```python
from build123d import *

# Parameters (mm, degrees)
SKETCH1_W           = 31.75
SKETCH1_H           = 7.9375
BOSS_EXTRUDE1_DEPTH = 3.175
SKETCH2_R           = 2.38125
BOSS_EXTRUDE2_DEPTH = 1.5875
SHELL1_T            = -1.5875
SKETCH3_R           = 1.5875
SKETCH3_R_2         = 0.79375
BOSS_EXTRUDE4_DEPTH = 1.397


with BuildPart() as part:
    # Sketch1 → Boss-Extrude1 (new body)
    with BuildSketch(Plane(origin=(0, 0, 0), x_dir=(1, 0, 0), z_dir=(0, 1, 0))):
        with Locations((15.875, 3.96875)):
            Rectangle(SKETCH1_W, SKETCH1_H)
    extrude(amount=BOSS_EXTRUDE1_DEPTH)

    # Sketch2 → Boss-Extrude2 (add)
    with BuildSketch(Plane(origin=(0, 3.175, 0), x_dir=(1, 0, 0), z_dir=(0, 1, 0))):
        with Locations((3.96875, 3.96875)):
            Circle(SKETCH2_R)
        with Locations((11.90625, 3.96875)):
            Circle(SKETCH2_R)
        with Locations((19.84375, 3.96875)):
            Circle(SKETCH2_R)
        with Locations((27.78125, 3.96875)):
            Circle(SKETCH2_R)
    extrude(amount=BOSS_EXTRUDE2_DEPTH)

    # Shell1
    shell1_openings = [part.faces().sort_by_distance(p)[0] for p in [
        (15.875, 0, -3.96875),
    ]]
    offset(amount=SHELL1_T, openings=shell1_openings, kind=Kind.INTERSECTION)

    # Sketch3 → Boss-Extrude4 (add)
    with BuildSketch(Plane.XZ.offset(-1.5875)):
        with Locations((7.540625, -3.96875)):
            Circle(SKETCH3_R)
        with Locations((7.540625, -3.96875)):
            Circle(SKETCH3_R_2, mode=Mode.SUBTRACT)
        with Locations((15.478125, -3.96875)):
            Circle(SKETCH3_R)
        with Locations((15.478125, -3.96875)):
            Circle(SKETCH3_R_2, mode=Mode.SUBTRACT)
        with Locations((23.415625, -3.96875)):
            Circle(SKETCH3_R)
        with Locations((23.415625, -3.96875)):
            Circle(SKETCH3_R_2, mode=Mode.SUBTRACT)
    extrude(amount=BOSS_EXTRUDE4_DEPTH)


solid = part.part
```
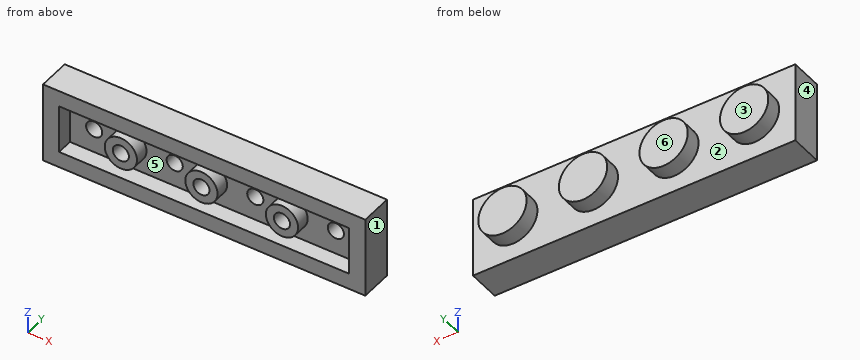
For this review, take the finished solid that the model builds, in its own axes (mm). Face numbers are marked on the shaded views. A direction names the side the tool comes from. Round coordinates to 2 decimals unless told otherwise and drop trailing zeros. Write each question's results on one line, items separated by ' | '.
Item 1: To check wall thickness, follow line 1 along Z through (x, y) = (29, 0.55); line 2 along X through (y, z) = (0.6, -2.25); line 3 along X through (y, z) = (4.2, -6). State the ranges of each line that lie inside material, in increasing order. Write a range as from..to.
Calculated:
line 1: z = -7.94..-6.35, -1.59..0 | line 2: x = 0..1.59, 30.16..31.75 | line 3: x = 2.73..5.21, 10.66..13.15, 18.6..21.09, 26.54..29.02
Item 2: Take a section at A-A on y = 0.6. Count the separate pieces of the cut face and the enclosed holes in it, then the cut area to 3 significant figures.
Calculated:
separate pieces: 4 | enclosed holes: 4 | area: 134 mm^2
Item 3: For the marked faces 5 and 6, list the 3-axis set-ups (+Z, -Z, +X, -X, +Y, -Y) from which the entire face can be reached by the end or side of a thin tool; tool diameter is ignored.
Calculated:
face 5: -Y | face 6: +Z, -Z, +X, -X, +Y
Item 4: Draft analysis for pull direction X (two halves, no side actions). For the marked faces 1, 2, 3 and 4, state which applies: pulls with the +X half, pulls with the -X half, needs draft (parallel to the pull), parting line crosses it, or undercut.
Calculated:
face 1: pulls with the +X half | face 2: undercut | face 3: needs draft | face 4: pulls with the -X half
Item 5: For pin 1 (1.4 mm diameter, centred on x = 14, z = -5, fed in from -Y); pin 2 (1.3 mm diameter, centred on x = 27.78, z = -3.97, fed in from -Y) (3 decimals); pin 3 (1.7 mm diameter, centred on x = 3.5, z = -4, fed in from -Y), all flat-tipped, find the tip position at first contact; note any pin that passes through.
Calculated:
pin 1: stops at y = 0.19 | pin 2: stops at y = 3.175 | pin 3: stops at y = 1.59
